Geometry check sheet. Reference: the model listing, model coordinates, mm. A direction names the side the tool comes from. Give positions to 0.01 mm unless a question says otherwise; leave off trailing zeros. Loops run counter-clockwise (first coordinate to the right, second up) from the corner with the lowest first, then second, coordinate; pieces in that order, holes last. Notation, with made-up numbers: (71.25, 23) - (90.25, 23) arc R18 cw to (90.25, 35) - close; hole circle Ø8 at (33.5, 32.25). An arc over 180 degrees is marked (long way). Use a Markdown table: item, result. Add a question column.
1. Cross-section at D-D on z = -3.5. Enter the section's corners in (x, y).
2. Cross-section at C-C on y = 0.45. Enter the section's corners in (x, z) (3 decimals).
3. Set-up check for faces 1 (the flat face through (1.98, 2.8, -3.43)), 2 (the cylindrical face through (4.041, 0.394, -5.217)), 3 (the flat face through (3, 3, -4)): record each of +Z, -Z, +X, -X, +Y, -Y from which the full face is reachable in a straight line by a thin tool's end or side.
4. Cross-section at B-B on x = 3.5. Enter the section's corners in (y, z).
5. Draft check along Z on faces 4 (the flat face through (6.655, 1.479, -3.451)), 5 (the flat face through (3.451, 1.521, -6.645)), 6 (the flat face through (3.451, 1.479, -0.345)), 7 (the flat face through (4, 0.8, -3)). Enter one of: pulls with the +Z half, pulls with the -Z half, needs draft (parallel to the pull), parting line crosses it, or undercut.
6. Material ranges on L1, parallel to Y at x = 4, z = -4; L2, parallel to Z at x = 5.25, y = 2.7; L3, parallel to Z at x = 2, y = 2.2, recorded low to high.
7. Depth check by flat-ended pin: P1, Ø1.5, axis at y = 2.5, z = -1, coming from the +X side; P2, Ø1.8, axis at x = 3.5, z = -4, coming from the -Y side. Enter the tip coordinate at first touch or a pass-through.
8. Cross-section at A-A on z = -1.5. Enter the section's corners in (x, y), and give its area (3 significant figures).
from build123d import *

# Parameters (mm, degrees)
SKETCH1_W           = 7
SKETCH1_H           = 7
BOSS_EXTRUDE1_DEPTH = 3
CUT_EXTRUDE1_DEPTH  = 7
CUT_EXTRUDE2_DEPTH  = 11
SKETCH4_R           = 1.8
CUT_EXTRUDE3_DEPTH  = 0.8
SKETCH5_W           = 1.947102418
SKETCH5_H           = 1.1
SKETCH5_W_2         = 1.102897582
SKETCH5_H_2         = 3.4
CUT_EXTRUDE4_DEPTH  = 0.4


with BuildPart() as part:
    # Sketch1 → Boss-Extrude1 (new body)
    with BuildSketch(Plane(origin=(0, 0, 0), x_dir=(1, 0, 0), z_dir=(0, 1, 0))):
        with Locations((3.5, 3.5)):
            Rectangle(SKETCH1_W, SKETCH1_H)
    extrude(amount=BOSS_EXTRUDE1_DEPTH)

    # Sketch2 → Cut-Extrude1 (cut)
    with BuildSketch(Plane.XY):
        Polygon((0, 0), (0.7, 3), (0, 3), align=None)
        Polygon((7, 0), (6.3, 3), (7, 3), align=None)
    extrude(amount=-CUT_EXTRUDE1_DEPTH, mode=Mode.SUBTRACT)

    # Sketch3 → Cut-Extrude2 (cut)
    with BuildSketch(Plane(origin=(0, 0, 0), x_dir=(0, 0, -1), z_dir=(1, 0, 0))):
        Polygon((0, 0), (0.7, 3), (0, 3), align=None)
        Polygon((7, 3), (6.3, 3), (7, 0), align=None)
    extrude(amount=CUT_EXTRUDE2_DEPTH, mode=Mode.SUBTRACT)

    # Sketch4 → Cut-Extrude3 (cut)
    with BuildSketch(Plane.XZ):
        with Locations(Location((3.5, -3.5, 0), (0, 0, 270))):
            Circle(SKETCH4_R)
    extrude(amount=-CUT_EXTRUDE3_DEPTH, mode=Mode.SUBTRACT)

    # Sketch5 → Cut-Extrude4 (cut)
    with BuildSketch(Plane(origin=(0, 3, 0), x_dir=(1, 0, 0), z_dir=(0, 1, 0))):
        Polygon((1.3, 2.75), (2.65, 1.4), (2.65, 2.2), (2.65, 3.3), (2.65, 4.1), align=None)
        with Locations((3.623551209, 2.75)):
            Rectangle(SKETCH5_W, SKETCH5_H)
        with Locations((5.148551209, 3.9)):
            Rectangle(SKETCH5_W_2, SKETCH5_H_2)
    extrude(amount=-CUT_EXTRUDE4_DEPTH, mode=Mode.SUBTRACT)


solid = part.part
Values found:
| question | item | result |
|---|---|---|
| 1 | outline | (0, 0) - (1.7, 0) - (1.7, 0.8) - (5.3, 0.8) - (5.3, 0) - (7, 0) - (6.3, 3) - (5.7, 3) - (5.7, 2.6) - (4.6, 2.6) - (4.6, 3) - (2.65, 3) - (2.65, 2.6) - (2.05, 2.6) - (2.05, 3) - (0.7, 3) - close |
| 2 | outline | (0.105, -6.895) - (6.895, -6.895) - (6.895, -0.105) - (0.105, -0.105) - close; hole circle Ø3.6 at (3.5, -3.5) |
| 3 | face 1 | +Y |
| 3 | face 2 | -Y |
| 3 | face 3 | +Z, -Z, +X, -X, +Y |
| 4 | outline | (0, -7) - (3, -6.3) - (3, -3.3) - (2.6, -3.3) - (2.6, -2.2) - (3, -2.2) - (3, -0.7) - (0, 0) - (0, -1.7) - (0.8, -1.7) - (0.8, -5.3) - (0, -5.3) - close |
| 5 | face 4 | needs draft |
| 5 | face 5 | pulls with the -Z half |
| 5 | face 6 | pulls with the +Z half |
| 5 | face 7 | undercut |
| 6 | L1 | y = 0.8 to 3 |
| 6 | L2 | z = -6.37 to -5.6, -2.2 to -0.63 |
| 6 | L3 | z = -6.49 to -0.51 |
| 7 | P1 | stops at x = 6.59 |
| 7 | P2 | stops at y = 0.8 |
| 8 | outline | (0, 0) - (7, 0) - (6.3, 3) - (2.65, 3) - (2.65, 2.6) - (2.55, 2.6) - (2.55, 3) - (0.7, 3) - close |
| 8 | area | 18.9 mm2 |
